Can you work these out from the model? Positions are in its coordinate system, mm. Face numbers are marked on the shaded views. A direction names the side the tool comes from. Round coordinates to 2 decimals unless told otherwise and drop trailing zeros. Write each loop counter-clockwise with the first axis right and the second up, starting at its lowest first coordinate (ties: lowest second). Pieces come first, ordered by that corner, then holes. Notation, with made-up numbers: M -11.5,0 L 13.5,0 A22 ccw 13.5,29 Z; hole C 53.25,78 d3. An arc over 180 degrees is marked long. Answer in a Markdown table with one row per item. Add a question column.
(1) I'm going to push flat-ended pins straight in: pin 1 (8.5 mm diameter, centred on y = -12.5, z = 16, fed in from -X) (3 decimals); pin 2 (1 mm diameter, centred on x = -21, z = 42.5, fed in from +Y); pin 3 (14.5 mm diameter, centred on x = 75.5, y = 2, fed in from -Z). Where does each tip first touch, or does it pass through?
(2) Suppose I cut it at C-C, the plane x = 102.5. Write out the boundary of the cut face in (y, z) (3 decimals).
(3) If I drill on probe 1 along Y at (x, z) = (-13, 37); probe 2 along Z at (x, y) = (-21, 37.5) (3 decimals); probe 3 along X at (y, z) = (50.5, -3.5) (3 decimals), over which ranges is the centre line in solid material (lowest first)?
(4) Suppose I cut it at A-A, the plane x = 63.5. Write out the boundary of the cut face in (y, z) (3 decimals), then the cut area to 3 significant figures.
(5) Suppose I cut it at B-B, the plane y = 37. Write out the boundary of the cut face in (x, z) (3 decimals), then the cut area to 3 significant figures.
(6) If we mould it in two halves opening along X, with no side actions, what happens to the marked faces 1, 2, 3 and 4? For each: released by +X, released by -X, zero draft, split by the parting line, or undercut.
(7) For the marked faces 5, 6, 7, 8 and 9, which set-ups out of +Z, -Z, +X, -X, +Y, -Y let a thin tool reach every point of the face, with its end or its side?
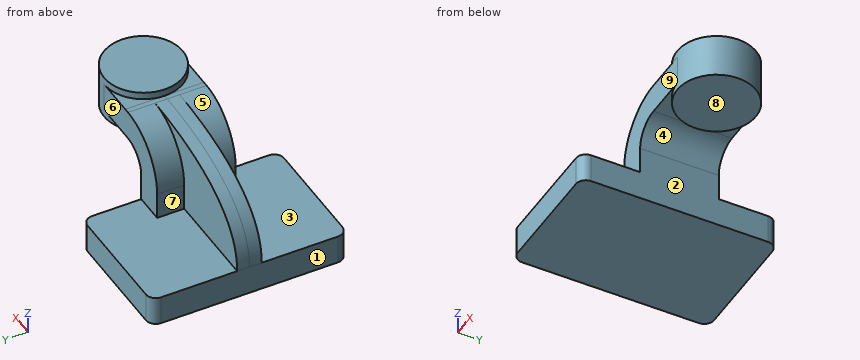
from build123d import *

# Parameters (mm, degrees)
F1_DEPTH = 63.5
F0_W     = 25.3999010601
F0_H     = 19.05
F2_DEPTH = 25.4
F3_DEPTH = 7.9375
F5_R     = 6.35


# Not quite as in the source:
# - ends of sketch curves that miss each other by under 0.0002 mm in the source are joined


with BuildPart() as f1:
    # F0 (on Front) → F1 (new body, symmetric)
    with BuildSketch(Plane.XZ):
        Polygon((22.225, 9.525), (-41.275, 9.525), (-41.275, -9.525), (41.275, -9.525), (41.275, 9.525), align=None)
    extrude(amount=F1_DEPTH, both=True)

    # F0 (on Front) → F2 (join, symmetric)
    with BuildSketch(Plane.XZ):
        with Locations((73.0249505301, 52.4002)):
            Rectangle(F0_W, F0_H)
        with BuildLine():
            Line((22.225, 27.0002), (22.225, 9.5249091869))
            Line((22.225, 9.5249091869), (41.275, 9.525))
            Line((41.275, 9.525), (41.275, 27.0002))
            ThreePointArc((41.275, 27.0002), (45.9246798487, 38.2255201513), (57.15, 42.8752))
            Line((57.15, 42.8752), (60.325, 42.8752))
            Line((60.325, 42.8752), (60.325, 61.9252))
            add(Edge.make_bspline(
                [(57.15, 61.9252), (59.3391618347, 61.9252), (59.4645664096, 61.9133971632), (60.325, 61.9252)],
                knots=[0.8556201459, 0.8556201459, 0.8556201459, 0.8556201459, 1, 1, 1, 1], degree=3))
            ThreePointArc((57.15, 61.9252), (32.4542956671, 51.6959043329), (22.225, 27.0002))
        make_face()
    extrude(amount=F2_DEPTH, both=True)

    # F0 (on Front) → F3 (join, symmetric)
    with BuildSketch(Plane.XZ):
        with BuildLine():
            add(Edge.make_bspline(
                [(-41.275, 9.525), (-41.2749116122, 61.5106898116), (44.1766459292, 61.9252), (57.15, 61.9252)],
                knots=[0, 0, 0, 0, 0.8556201459, 0.8556201459, 0.8556201459, 0.8556201459], degree=3))
            Line((-41.275, 9.525), (22.225, 9.525))
            Line((22.225, 9.525), (22.225, 27.0002))
            ThreePointArc((22.225, 27.0002), (32.4542956671, 51.6959043329), (57.15, 61.9252))
        make_face()
    extrude(amount=F3_DEPTH, both=True)

    # F0 (on Front) → F4 (revolve)
    with BuildSketch(Plane.XZ):
        Polygon((85.725, 66.675), (85.725, 61.9252), (85.725, 42.8752), (85.725, 38.1), (111.125, 38.1), (111.125, 66.675), align=None)
    revolve(axis=Axis((85.725, 0, 52.3875), (0, 0, 1)))

    # F5
    f5_edges = [f1.edges().sort_by_distance(p)[0] for p in [
        (41.275, -63.5, 0),
        (-41.275, -63.5, 0),
        (41.275, 63.5, 0),
        (-41.275, 63.5, 0),
    ]]
    fillet(f5_edges, radius=F5_R)


solid = f1.part
Calculated:
| question | item | result |
|---|---|---|
| 1 | pin 1 | x = 22.225 |
| 1 | pin 2 | y = 7.94 |
| 1 | pin 3 | z = 38.1 |
| 2 | outline | M -19.072,38.1 L 19.072,38.1 L 19.072,66.675 L -19.072,66.675 Z |
| 3 | probe 1 | -7.94 to 7.94 |
| 3 | probe 2 | -9.525 to 9.525 |
| 3 | probe 3 | -41.275 to 41.275 |
| 4 | outline | M -25.4,42.875 L -12.297,42.875 L -12.297,38.1 L 12.297,38.1 L 12.297,42.875 L 25.4,42.875 L 25.4,61.925 L 12.297,61.925 L 12.297,66.675 L -12.297,66.675 L -12.297,61.925 L -25.4,61.925 Z |
| 4 | area | 1,200 mm² |
| 5 | outline | M -41.275,-9.525 L 41.275,-9.525 L 41.275,9.525 L -41.275,9.525 Z |
| 5 | area | 1,570 mm² |
| 6 | face 1 | released by -X |
| 6 | face 2 | released by +X |
| 6 | face 3 | zero draft |
| 6 | face 4 | undercut |
| 7 | face 5 | +Z, -X, -Y |
| 7 | face 6 | +Z, +X, -X, +Y |
| 7 | face 7 | +Z, -X, +Y |
| 7 | face 8 | -Z, +X, +Y, -Y |
| 7 | face 9 | +Z, +X, -X, -Y |
